from build123d import *

# Parameters (mm, degrees)
F0_W     = 749.3
F0_H     = 749.3
F1_DEPTH = 19.05
F3_DEPTH = 114.3
F4_R     = 6.35
F5_DEPTH = 1.27
F6_R     = 6.35
F6_R_2   = 12.7
F6_R_3   = 38.1
F7_DEPTH = 25.4
F9_DEPTH = 37.592


with BuildPart() as f1:
    # F0 (on Top) → F1 (new body)
    with BuildSketch(Plane.XY):
        Rectangle(F0_W, F0_H)
    extrude(amount=F1_DEPTH)

    # F2 (on face) → F3 (cut)
    with BuildSketch(Plane.XY.offset(19.05)):
        Polygon((-352.425, 196.85), (-374.65, 219.075), (-374.65, -219.075), (-352.425, -196.85), align=None)
        Polygon((374.65, -219.075), (374.65, 219.075), (352.425, 196.85), (352.425, -196.85), align=None)
    extrude(amount=-F3_DEPTH, mode=Mode.SUBTRACT)

    # F4 (on face) → F5 (cut)
    with BuildSketch(Plane.XY.offset(19.05)):
        with Locations((0, 28.575)):
            Circle(F4_R)
        with Locations((-27.17644, 8.830161)):
            Circle(F4_R)
        with Locations((-16.795964, -23.117661)):
            Circle(F4_R)
        with Locations((16.795964, -23.117661)):
            Circle(F4_R)
        with Locations((27.17644, 8.830161)):
            Circle(F4_R)
    extrude(amount=-F5_DEPTH, mode=Mode.SUBTRACT)

    # F6 (on face) → F7 (cut)
    with BuildSketch(Plane.XY.offset(19.05)):
        with Locations((190.5, -317.5)):
            Circle(F6_R)
        with Locations((266.7, -317.5)):
            Circle(F6_R)
        with Locations((342.9, -317.5)):
            Circle(F6_R)
        with Locations((304.8, -289.56)):
            Circle(F6_R_2)
        with Locations((304.8, 289.56)):
            Circle(F6_R_2)
        with Locations((342.9, 317.5)):
            Circle(F6_R)
        with Locations((266.7, 317.5)):
            Circle(F6_R)
        with Locations((190.5, 317.5)):
            Circle(F6_R)
        with Locations((-304.8, -289.56)):
            Circle(F6_R_2)
        with Locations((-342.9, -317.5)):
            Circle(F6_R)
        with Locations((-266.7, -317.5)):
            Circle(F6_R)
        with Locations((-190.5, -317.5)):
            Circle(F6_R)
        with Locations((-190.5, 317.5)):
            Circle(F6_R)
        with Locations((-266.7, 317.5)):
            Circle(F6_R)
        with Locations((-342.9, 317.5)):
            Circle(F6_R)
        with Locations((-304.8, 289.56)):
            Circle(F6_R_2)
        with Locations((-139.7, 0)):
            Circle(F6_R_3)
        with Locations((139.7, 0)):
            Circle(F6_R_3)
    extrude(amount=-F7_DEPTH, mode=Mode.SUBTRACT)

    # F8 (on face) → F9 (cut)
    with BuildSketch(Plane(origin=(0, 0, 0), x_dir=(1, 0, 0), z_dir=(0, 0, -1))):
        with BuildLine():
            Line((-149.225, -374.65), (0, -374.65))
            Line((0, -374.65), (149.225, -374.65))
            Line((149.225, -374.65), (149.225, -287.42081))
            Line((149.225, -287.42081), (149.225, -286.705137))
            ThreePointArc((149.225, -286.705137), (0, -323.215), (-149.225, -286.705137))
            Line((-149.225, -286.705137), (-149.225, -287.42081))
            Line((-149.225, -287.42081), (-149.225, -374.65))
        make_face()
    extrude(amount=-F9_DEPTH, mode=Mode.SUBTRACT)


solid = f1.part
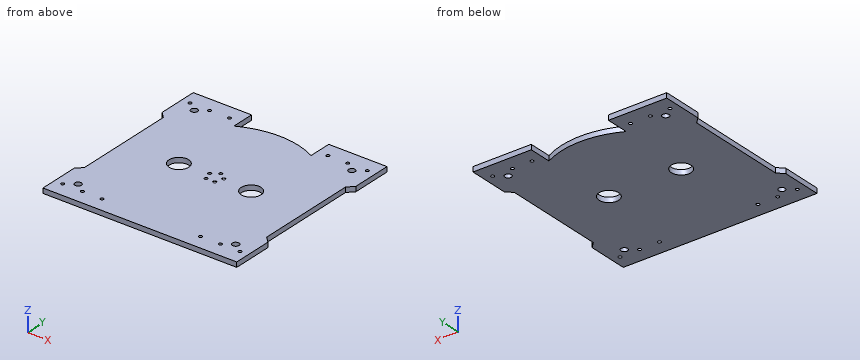
Geometry check sheet. Reference: the model listing, model coordinates, mm. Coordinates: 2 decimals unless noted, no trailing zeros. Write each loop counter-clockwise with the first axis right and the second up, starting at its lowest first coordinate (ties: lowest second). Pieces come first, ordered by that corner, then holes. Notation, with made-up numbers: (79, 75.25) -> (136, 75.25) arc R21 cw to (136, 86.25) -> close; hole circle Ø11 at (29, 18). An arc over 180 degrees is marked (long way). One line per question, with ' | ' between items.
1. Cross-section at A-A on x = 304.8. Record the cut outline in (y, z), and give its area (3 significant figures).
Answers:
outline: (-374.65, 0) -> (-302.26, 0) -> (-302.26, 19.05) -> (-374.65, 19.05) -> close; (-276.86, 0) -> (276.86, 0) -> (276.86, 19.05) -> (-276.86, 19.05) -> close; (302.26, 0) -> (374.65, 0) -> (374.65, 19.05) -> (302.26, 19.05) -> close | area: 13,300 mm²
2. Depth check by flat-ended pin: pin 1 Ø14.5 at (x, y) = (266.7, -317.5) entering from +Z; pin 2 Ø9.5 at (y, z) = (-74, 11) entering from -X (3 decimals); pin 3 Ø1.5 at (x, z) = (-120.5, 11) entering from +Y; pin 4 Ø4 at (y, z) = (21.5, 12.5) entering from +X (3 decimals). Enter the tip coordinate at first touch or a pass-through.
Answers:
pin 1: stops at z = 19.05 | pin 2: stops at x = -352.425 | pin 3: stops at y = 300.21 | pin 4: stops at x = 352.425
3. Cross-section at B-B on z = 9.5. State how many separate pieces and enclosed holes the cut face has, and give its area (3 significant figures).
Answers:
separate pieces: 1 | enclosed holes: 18 | area: 511,000 mm²
4. Thickness scan on probe 1 along Y at (x, z) = (-192, 15.25); probe 2 along Y at (x, z) = (-190.5, 8.25); probe 3 along X at (y, z) = (137, 5.5) (3 decimals). Record the ranges inside material, lowest first. Write a range as from..to.
Answers:
probe 1: y = -374.65..-323.67, -311.33..311.33, 323.67..374.65 | probe 2: y = -374.65..-323.85, -311.15..311.15, 323.85..374.65 | probe 3: x = -352.425..352.425
5. Cross-section at C-C on y = -154.5. Record the cut outline in (x, z) (3 decimals), and give its area (3 significant figures).
Answers:
outline: (-352.425, 0) -> (352.425, 0) -> (352.425, 19.05) -> (-352.425, 19.05) -> close | area: 13,400 mm²
